```python
from build123d import *

# Parameters (mm, degrees)
SKETCH_1_R               = 26
EXTRUDE_1_DEPTH          = 35
SKETCH_3_R               = 22.5
CUT_EXTRUDE_1_DEPTH      = 11
CUT_EXTRUDE_START        = -19
SKETCH_4_R               = 22.5
CUT_EXTRUDE_2_DEPTH      = 19
SKETCH_13_W              = 24
SKETCH_13_H              = 13
CUT_EXTRUDE_3_DEPTH      = 4
EXTRUDE_2_DEPTH          = 8
SKETCH_15_W              = 4
SKETCH_15_H              = 12
SKETCH_15_W_2            = 4.3
CUT_EXTRUDE_5_DEPTH      = 4
SKETCH_17_R              = 1
CUT_EXTRUDE_6_DEPTH      = 4
SKETCH_20_R              = 3
EXTRUDE_3_DEPTH          = 5
SKETCH_21_R              = 1
CUT_EXTRUDE_9_DEPTH      = 5
SKETCH_24_W              = 2.5
SKETCH_24_H              = 8
CUT_EXTRUDE_12_DEPTH     = 5
SKETCH_25_R              = 2
CUT_EXTRUDE_13_DEPTH     = 1
SKETCH_26_R              = 1
CUT_EXTRUDE_14_DEPTH     = 71.996321423
PATTERN_CIRCULAR_1_COUNT = 4
CHAMFER_1_SIZE           = 0.5


with BuildPart() as part:
    # Эскиз1 → Бобышка-Вытянуть1 (new body)
    with BuildSketch(Plane.XY):
        Circle(SKETCH_1_R)
    extrude(amount=EXTRUDE_1_DEPTH)

    # Эскиз3 → Вырез-Вытянуть1 (cut)
    with BuildSketch(Plane(origin=(0, 0, 0), x_dir=(-1, 0, 0), z_dir=(0, 0, -1))):
        Circle(SKETCH_3_R)
    extrude(amount=-CUT_EXTRUDE_1_DEPTH, mode=Mode.SUBTRACT)

    # Эскиз4 → Вырез-Вытянуть2 (cut)
    with BuildSketch(Plane.XY.offset(35).offset(CUT_EXTRUDE_START)):
        with Locations(Location((0, 0, 0), (0, 0, 180))):
            Circle(SKETCH_4_R)
    extrude(amount=CUT_EXTRUDE_2_DEPTH, mode=Mode.SUBTRACT)

    # Эскиз13 → Вырез-Вытянуть3 (cut)
    with BuildSketch(Plane.XY.offset(16)):
        with Locations((-5, 0)):
            Rectangle(SKETCH_13_W, SKETCH_13_H)
    extrude(amount=-CUT_EXTRUDE_3_DEPTH, mode=Mode.SUBTRACT)

    # Эскиз14 → Бобышка-Вытянуть2 (add)
    with BuildSketch(Plane.XY.offset(26.5)):
        with BuildLine():
            Line((14.2, -20.575713839), (14.2, 20.575713839))
            ThreePointArc((14.2, 20.575713839), (10.596324929, 22.643274896), (6.7, 24.0854728))
            Line((6.7, 24.0854728), (6.7, -24.0854728))
            ThreePointArc((6.7, -24.0854728), (10.596324929, -22.643274896), (14.2, -20.575713839))
        make_face()
        with BuildLine():
            Line((-17.5, -17.853571071), (-17.5, 17.853571071))
            ThreePointArc((-17.5, 17.853571071), (-25, 0), (-17.5, -17.853571071))
        make_face()
    extrude(amount=EXTRUDE_2_DEPTH)

    # Эскиз15 → Вырез-Вытянуть5 (cut)
    with BuildSketch(Plane.XY.offset(34.5)):
        with Locations((-19.5, 0)):
            Rectangle(SKETCH_15_W, SKETCH_15_H)
        with Locations((8.85, 0)):
            Rectangle(SKETCH_15_W_2, SKETCH_15_H)
    extrude(amount=-CUT_EXTRUDE_5_DEPTH, mode=Mode.SUBTRACT)

    # Эскиз17 → Вырез-Вытянуть6 (cut)
    with BuildSketch(Plane.XY.offset(30.5)):
        with Locations((-19.1, 0)):
            Circle(SKETCH_17_R)
        with Locations((8.6, 0)):
            Circle(SKETCH_17_R)
    extrude(amount=-CUT_EXTRUDE_6_DEPTH, mode=Mode.SUBTRACT)

    # Эскиз20 → Бобышка-Вытянуть3 (add)
    with BuildSketch(Plane.XY.offset(35)):
        with Locations((-15.556349186, 15.556349186)):
            Circle(SKETCH_20_R)
        with Locations((15.556349186, 15.556349186)):
            Circle(SKETCH_20_R)
        with Locations((15.556349186, -15.556349186)):
            Circle(SKETCH_20_R)
        with Locations((-15.556349186, -15.556349186)):
            Circle(SKETCH_20_R)
    extrude(amount=-EXTRUDE_3_DEPTH)

    # Эскиз21 → Вырез-Вытянуть9 (cut)
    with BuildSketch(Plane.XY.offset(35)):
        with Locations((-15.556349186, 15.556349186)):
            Circle(SKETCH_21_R)
        with Locations((15.556349186, 15.556349186)):
            Circle(SKETCH_21_R)
        with Locations((15.556349186, -15.556349186)):
            Circle(SKETCH_21_R)
        with Locations((-15.556349186, -15.556349186)):
            Circle(SKETCH_21_R)
    extrude(amount=-CUT_EXTRUDE_9_DEPTH, mode=Mode.SUBTRACT)

    # Эскиз24 → Вырез-Вытянуть12 (cut)
    with BuildSketch(Plane.XY.offset(16)):
        with Locations((12.25, 0)):
            Rectangle(SKETCH_24_W, SKETCH_24_H)
    extrude(amount=-CUT_EXTRUDE_12_DEPTH, mode=Mode.SUBTRACT)

    # Эскиз25 → Вырез-Вытянуть13 (cut)
    with BuildSketch(Plane(origin=(-18.384776311, -18.384776311, 35), x_dir=(-0.7071067811865678, 0.7071067811865273, 0), z_dir=(-0.7071067811865273, -0.7071067811865678, 0))):
        with Locations(Location((0, 30, 0), (0, 0, 180))):
            Circle(SKETCH_25_R)
    cut_extrude_13 = extrude(amount=-CUT_EXTRUDE_13_DEPTH, mode=Mode.SUBTRACT)

    # Эскиз26 → Вырез-Вытянуть14 (cut, through all)
    with BuildSketch(Plane(origin=(-17.67766953, -17.67766953, 0), x_dir=(0, 0, 1), z_dir=(-0.7071067811865273, -0.7071067811865678, 0))):
        with Locations(Location((5, 0, 0), (0, 0, 270))):
            Circle(SKETCH_26_R)
    cut_extrude_14 = extrude(amount=-CUT_EXTRUDE_14_DEPTH, mode=Mode.SUBTRACT)

    # Круговой массив1: Вырез-Вытянуть13, Вырез-Вытянуть14 ×4 about axis
    pattern_circular_1_axis = Axis((0, 0, 0), (0, 0, 1))
    add([cut_extrude_13.rotate(pattern_circular_1_axis, i * 360 / PATTERN_CIRCULAR_1_COUNT) for i in range(1, PATTERN_CIRCULAR_1_COUNT)], mode=Mode.SUBTRACT)
    add([cut_extrude_14.rotate(pattern_circular_1_axis, i * 360 / PATTERN_CIRCULAR_1_COUNT) for i in range(1, PATTERN_CIRCULAR_1_COUNT)], mode=Mode.SUBTRACT)

    # Фаска1
    chamfer_1_edges = [part.edges().sort_by_distance(p)[0] for p in [
        (22.5, 0, 0),
    ]]
    chamfer(chamfer_1_edges, length=CHAMFER_1_SIZE)


solid = part.part
```
Check sheet for the modelled part. Datum: model origin and axes. Units: mm. A direction names the side the tool comes from. Coordinates: 2 decimals unless noted, no trailing zeros. Order: outer loops, then holes, each group sorted by start corner. A loop starts at its lowest first (then second) coordinate and runs counter-clockwise, first axis right, second up. Notation, with made-up numbers: M 2.25,-30.75 L 40.25,-30.75 A26 cw 40.25,8.25 Z; hole C 54,73.5 d5. An arc over 180 degrees is marked long. One line per question, with ' | ' between items. Start each with the question number.
Item 1: Gauge pin test, flat ends, axial feed: P1, Ø10, axis at x = 13, z = 27.5, coming from the -Y side; P2, Ø6, axis at y = 19.5, z = 18.5, coming from the -X side; P3, Ø4, axis at x = -19, y = 5.5, coming from the +Z side. Record the tip position at first contact, or that the pin passes through.
Item 2: Sectioned sample at B-B on z = 23. Record the cut outline in (x, y).
Item 3: Sectioned sample at C-C on y = 0. Count the separate pieces of the cut face and the enclosed holes in it, and give its area (3 significant figures).
Item 4: Material ranges on line 1 (Y direction, x = 0, z = 8.5); line 2 (Z direction, x = 13, y = 9.5); line 3 (Z direction, x = -20, y = -4.5), recorded low to high.
Item 5: Mould release check, pull along Z, two halves, no side actions. Record for faces 1 (the cylindrical face through (18, 18, 7)), 2 (the flat face through (13.5, 0, 14)), 3 (the flat face through (0, 0, 11)): pulls with the +Z half, pulls with the -Z half, needs draft (parallel to the pull), parting line crosses it, or undercut.
Item 6: Sectioned sample at A-A on x = 0. Record the cut outline in (y, z), and give its area (3 significant figures).
Item 7: Access from +Z, -Z, +X, -X, +Y, -Y to the whole of each face (thin tool, end or side, straight path). Record for faces 4 (the flat face through (-14, 14, 35)), 5 (the cylindrical face through (22.48, -0.99, 25.37)), 6 (the flat face through (-20, -6, 33)).
Answer below:
1) P1: stops at y = -24.74 | P2: stops at x = -20.09 | P3: stops at z = 34.5
2) outline: C 0,0 d52; hole C 0,0 d45
3) separate pieces: 5 | enclosed holes: 0 | area: 412 mm^2
4) line 1: y = -26 to -22.5, 22.5 to 26 | line 2: z = 11 to 16, 26.5 to 34.5 | line 3: z = 11 to 16, 26.5 to 30.5
5) face 1: undercut | face 2: needs draft | face 3: pulls with the -Z half
6) outline: M -26,0 L -23,0 L -22.5,0.5 L -22.5,11 L 22.5,11 L 22.5,0.5 L 23,0 L 26,0 L 26,35 L 22.5,35 L 22.5,16 L 6.5,16 L 6.5,12 L -6.5,12 L -6.5,16 L -22.5,16 L -22.5,35 L -26,35 Z | area: 418 mm^2
7) face 4: +Z, +X, -X, +Y, -Y | face 5: none | face 6: +Z
